```python
from build123d import *

# Parameters (mm, degrees)
SKETCH1_W           = 3
SKETCH1_H           = 6
BOSS_EXTRUDE1_DEPTH = 3.175


with BuildPart() as part:
    # Sketch1 → Boss-Extrude1 (new body)
    with BuildSketch(Plane.XY):
        Polygon((0, 120), (-3.175, 120), (-3.175, 98.54), (0, 98.54), (0, 73.905), (-3.175, 73.905), (-3.175, 49.27), (0, 49.27), (0, 24.635), (-3.175, 24.635), (-3.175, 0), (0, 0), (0, -3.175), (33.358811077, -3.175), (33.358811077, 0), (66.692144411, 0), (66.692144411, -3.175), (100, -3.175), (100, 0), (103.175, 0), (103.175, 24.635), (100, 24.635), (100, 49.27), (103.175, 49.27), (103.175, 73.905), (100, 73.905), (100, 98.54), (103.175, 98.54), (103.175, 120), (100, 120), (100, 123.175), (66.666666667, 123.175), (66.666666667, 120), (33.333333333, 120), (33.333333333, 123.175), (0, 123.175), align=None)
        with Locations((98.5, 60)):
            Rectangle(SKETCH1_W, SKETCH1_H, mode=Mode.SUBTRACT)
        Polygon((3.024208093, 62.980047574), (3.026755867, 56.980048114), (0.026756138, 56.978774227), (0.024208364, 62.978773686), align=None, mode=Mode.SUBTRACT)
    extrude(amount=BOSS_EXTRUDE1_DEPTH)


solid = part.part
```
Input: part model. Units: mm. Frame: model coordinates. A direction names the side the tool comes from. Round coordinates to 2 decimals unless told otherwise and drop trailing zeros. Loops run counter-clockwise (first coordinate to the right, second up) from the corner with the lowest first, then second, coordinate; pieces in that order, holes last. Notation, with made-up numbers: (-22.75, 1.25) - (30.25, 1.25) arc R18 ccw to (30.25, 34.25) - close; hole circle Ø5 at (16.5, -19). An arc over 180 degrees is marked (long way). One line per item, written item: value. Start each with the question number.
(1) Access query for faces 4 (the flat face through (100, 37, 2)), 5 (the flat face through (66.667, 122, 2)), 6 (the flat face through (0, -2, 2)), 7 (the flat face through (-2, 73.905, 2)), 8 (the flat face through (0, 122, 2)). Directions: +Z, -Z, +X, -X, +Y, -Y. A direction counts if a zero-diameter tool reaches every point of the face in a straight line with its end or side. Return the directions, or none.
(2) Ray query, line 1 (Y direction, x = 2, z = 0.25) (3 decimals); line 2 (Y direction, x = 42, z = 0.2); line 3 (X direction, y = 94, z = 2.75). Return the intervals inside material, ascending. Write a range as [from, to].
(3) Section C-C, the plane x = 61. Return loops of the section in (y, z) (3 decimals).
(4) Section B-B, the plane y = 44. Return loops of the section in (x, z) (3 decimals), plus the area to 4 significant figures.
(5) Section A-A, the plane z = 2.4. Count the separate pieces of the cut face and the enclosed holes in it, plus the area to 3 significant figures.
(6) Draft query along Y for faces 1 (the flat face through (-3.175, 109, 2)), 2 (the flat face through (102, 120, 2)), 3 (the flat face through (-2, 24.635, 2)). Return one class per face: +Y half, -Y half, draft (parallel to the pull), parting line (faces both ways), or undercut.
(7) Contact query for flat-ended pins moving along their axis: P1, Ø1, axis at x = 102.5, z = 2, coming from the -Y side; P2, Ø1.6, axis at y = 82.5, z = 1, coming from the -X side; P3, Ø1.6, axis at y = -2, z = 1.5, coming from the +X side. Output: stop coordinate, or through.
Results below:
1. face 4: +Z, -Z, +X
1. face 5: +Z, -Z, +Y
1. face 6: +Z, -Z, -X, -Y
1. face 7: +Z, -Z, -X
1. face 8: +Z, -Z, -X, +Y
2. line 1: [-3.175, 56.98], [62.98, 123.175]
2. line 2: [0, 120]
2. line 3: [0, 100]
3. outline: (0, 0) - (120, 0) - (120, 3.175) - (0, 3.175) - close
4. outline: (0, 0) - (100, 0) - (100, 3.175) - (0, 3.175) - close
4. area: 317.5 mm^2
5. separate pieces: 1
5. enclosed holes: 2
5. area: 12,800 mm^2
6. face 1: draft
6. face 2: +Y half
6. face 3: undercut
7. P1: y = 0
7. P2: x = 0
7. P3: x = 100
